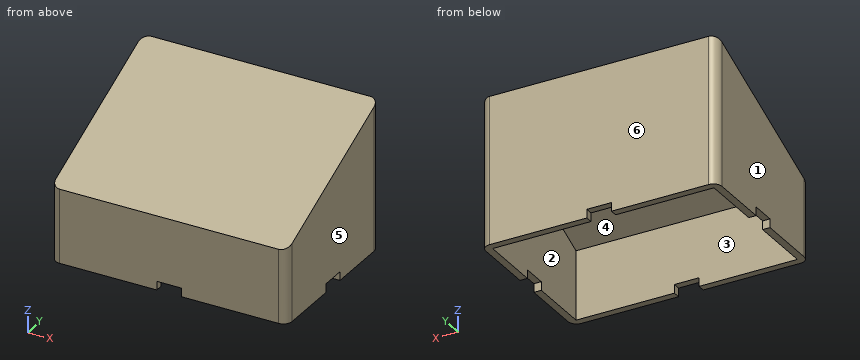
```python
from build123d import *

# Parameters (mm, degrees)
CROQUIS1_W              = 96
CROQUIS1_H              = 66
SALIENTE_EXTRUIR1_DEPTH = 60
CORTAR_EXTRUIR1_DEPTH   = 100
VACIADO1_T              = -3
CROQUIS3_W              = 3
CROQUIS3_H              = 5
CROQUIS3_W_2            = 5
CROQUIS3_H_2            = 3
CROQUIS3_W_3            = 10
CROQUIS3_H_3            = 10
CORTAR_EXTRUIR2_DEPTH   = 3.5
REDONDEO1_R             = 3.5


with BuildPart() as part:
    # Croquis1 → Saliente-Extruir1 (new body)
    with BuildSketch(Plane.XY):
        with Locations((48, 33)):
            Rectangle(CROQUIS1_W, CROQUIS1_H)
    extrude(amount=SALIENTE_EXTRUIR1_DEPTH)

    # Croquis2 → Cortar-Extruir1 (cut)
    with BuildSketch(Plane(origin=(96, 0, 0), x_dir=(0, 0, -1), z_dir=(1, 0, 0))):
        Polygon((-60, 66), (-30, 0), (-60, 0), align=None)
    extrude(amount=-CORTAR_EXTRUIR1_DEPTH, mode=Mode.SUBTRACT)

    # Vaciado1
    vaciado1_openings = [part.faces().sort_by_distance(p)[0] for p in [
        (48, 33, 0),
    ]]
    offset(amount=VACIADO1_T, openings=vaciado1_openings, kind=Kind.INTERSECTION)

    # Croquis3 → Cortar-Extruir2 (cut)
    with BuildSketch(Plane(origin=(0, 0, 0), x_dir=(-1, 0, 0), z_dir=(0, 0, -1))):
        with Locations((-1.5, 35.5)):
            Rectangle(CROQUIS3_W, CROQUIS3_H)
        with Locations((-1.5, 30.5)):
            Rectangle(CROQUIS3_W, CROQUIS3_H)
        with Locations((-45.5, 64.5)):
            Rectangle(CROQUIS3_W_2, CROQUIS3_H_2)
        with Locations((-50.5, 64.5)):
            Rectangle(CROQUIS3_W_2, CROQUIS3_H_2)
        with Locations((-48, 1.5)):
            Rectangle(CROQUIS3_W_3, CROQUIS3_H_2)
        with Locations((-94.5, 33)):
            Rectangle(CROQUIS3_W, CROQUIS3_H_3)
    extrude(amount=-CORTAR_EXTRUIR2_DEPTH, mode=Mode.SUBTRACT)

    # Redondeo1
    redondeo1_edges = [part.edges().sort_by_distance(p)[0] for p in [
        (96, 0, 15),
        (0, 0, 15),
        (0, 66, 30),
        (96, 66, 30),
    ]]
    fillet(redondeo1_edges, radius=REDONDEO1_R)


solid = part.part
```
CAD build for the part. Positions are in the model's coordinates, mm. Face numbers are marked on the shaded views. A direction names the side the tool comes from. Coordinates: 2 decimals unless noted, no trailing zeros. Loops run counter-clockwise (first coordinate to the right, second up) from the corner with the lowest first, then second, coordinate; pieces in that order, holes last. Notation, with made-up numbers: (19, 74) - (25, 74) arc R29 ccw to (25, 110) - close; hole circle Ø11 at (-9, -24). An arc over 180 degrees is marked (long way). Return JSON: item names as keys, results as strings.
1. Band-saw the part on D-D (z = 53). Give the cut face in (x, y).
Result:
{"outline": "(0, 50.6) - (96, 50.6) - (96, 62.5) arc R3.5 ccw to (92.5, 66) - (3.5, 66) arc R3.5 ccw to (0, 62.5) - close; hole (3, 57.85) - (93, 57.85) - (93, 63) - (3, 63) - close"}
2. Band-saw the part on B-B (x = 41). Give the cut face in (y, z).
Result:
{"outline": "(0, 0) - (3, 0) - (3, 28.07) - (63, 55.34) - (63, 0) - (66, 0) - (66, 60) - (0, 30) - close"}
3. Band-saw the part on C-C (y = 36). Give the cut face in (x, z).
Result:
{"outline": "(0, 3.5) - (3, 3.5) - (3, 43.07) - (93, 43.07) - (93, 3.5) - (96, 3.5) - (96, 46.36) - (0, 46.36) - close"}
4. 3-axis set-ups, long thin cutter, end or side, ignore diameter. For the marked faces 1 and 2: which of +Z, -Z, +X, -X, +Y, -Y reach the whole face in a straight line?
Result:
{"face 1": "+Z, -Z, -X, +Y, -Y", "face 2": "-Z"}
5. Drop flat-ended pins along their axis: pin 1 (6 mm diameter, centred on x = 48.5, z = 39, fed in from -Y); pin 2 (2.5 mm diameter, centred on y = 1.5, z = 1.5, fed in from +X); pin 3 (5 mm diameter, centred on x = 51.5, y = 47, fed in from +Z). Give the stop position or say it passes through.
Result:
{"pin 1": "stops at y = 13.2", "pin 2": "stops at x = 95.92", "pin 3": "stops at z = 52.5"}
6. Probe L1, parallel to Y at x = 31, z = 25; L2, parallel to X at y = 53.5, z = 5.5; L3, parallel to Y at x = 15, z = 48.5. List the from-to ranges inside material, lowest first. Write a range as from..to.
Result:
{"L1": "y = 0..3, 63..66", "L2": "x = 0..3, 93..96", "L3": "y = 40.7..47.95, 63..66"}
7. Band-saw the part on A-A (z = 20). Give the cut face in (x, y), and give its area (3 significant figures).
Result:
{"outline": "(0, 3.5) arc R3.5 ccw to (3.5, 0) - (92.5, 0) arc R3.5 ccw to (96, 3.5) - (96, 62.5) arc R3.5 ccw to (92.5, 66) - (3.5, 66) arc R3.5 ccw to (0, 62.5) - close; hole (3, 3) - (93, 3) - (93, 63) - (3, 63) - close", "area": "925 mm2"}
8. Mould opens along X. For the marked faces 3, 4, 5 and 6 say: released by +X, released by -X, zero draft, split by the parting line, or undercut.
Result:
{"face 3": "undercut", "face 4": "undercut", "face 5": "released by +X", "face 6": "zero draft"}
